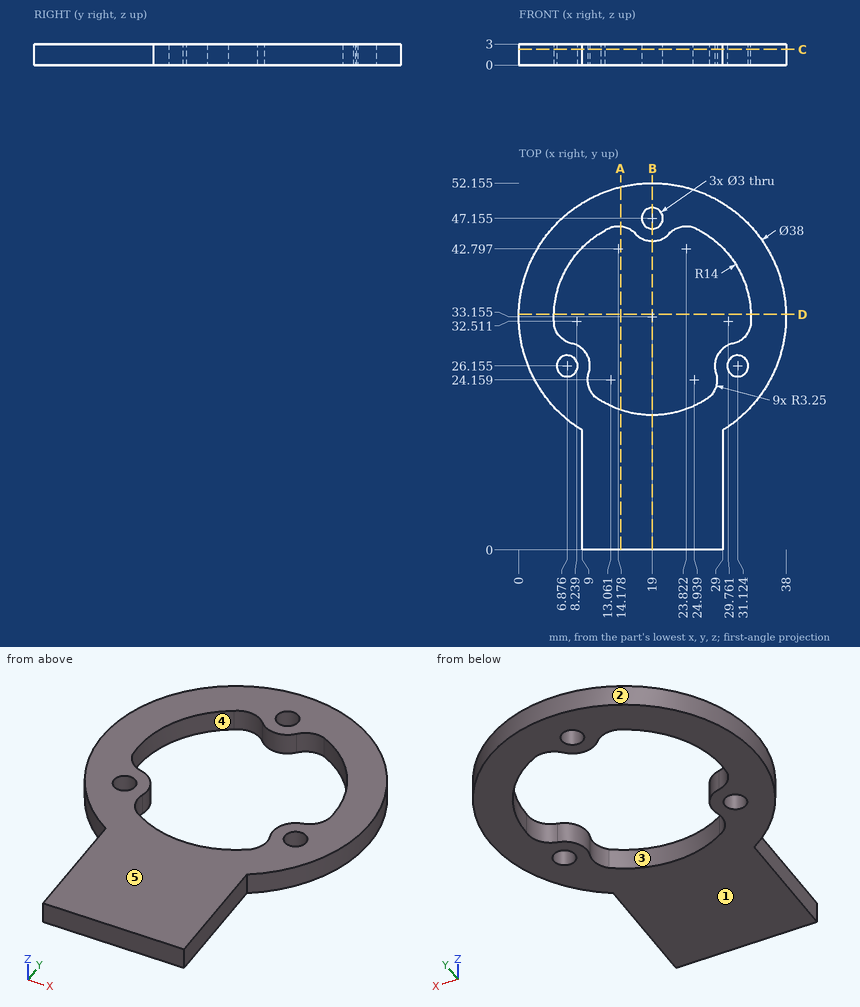
Can you work these out from the drawing? Everything is in mm from the part's minimum corner. A direction names the side the tool comes from. Give positions to 0.01 mm unless a question says otherwise; leave off trailing zeros. Order: outer loops, then holes, each group sorted by start corner. A loop starts at its lowest first (then second) coordinate and runs counter-clockwise, first axis right, second up.
1. Suppose I cut it at C-C (z = 2.25). Give the number of separate pieces and of enclosed holes in the cut face, plus the area to 3 significant figures.
2. Suppose I cut it at A-A (x = 14.5). List the corners of the cut face in (y, z) for me (1 decimal).
3. For the marked faces 4 and 5, which set-ups out of +Z, -Z, +X, -X, +Y, -Y let a thin tool reach every point of the face, with its end or its side?
4. I need wall thicknesses on L1, parallel to Y at x = 19, z = 2.15 (1 decimal); L2, parallel to Y at x = 30.5, z = 1.9 (1 decimal); L3, parallel to X at y = 4, z = 1.2. Which ranges of each line are inside material? Lowest first, please.
5. Suppose I cut it at B-B (x = 19). List the corners of the cut face in (y, z) for me (1 decimal).
6. Will these pins go through, and if not, where does the flat tip stop? P1, Ø1.5, axis at y = 7.5, z = 1.5, coming from the -X side; P2, Ø1.5, axis at y = 4.5, z = 1.5, coming from the +X side; P3, Ø1, axis at x = 14, z = 1.5, coming from the +Y side (1 decimal).
7. We'd pull the mould along X, two halves only. Please class the marked faces 1, 2 and 3: pulls with the +X half, pulls with the -X half, needs draft (parallel to the pull), parting line crosses it, or undercut.
8. Suppose I cut it at D-D (y = 33.5). List the corners of the cut face in (x, z) for me (1 decimal).
Solved:
1. separate pieces: 1
1. enclosed holes: 4
1. area: 854 mm2
2. outline: (0, 0) - (19.9, 0) - (19.9, 3) - (0, 3) - close; (46, 0) - (51.6, 0) - (51.6, 3) - (46, 3) - close
3. face 4: +Z, -Z
3. face 5: +Z, +X, -X, +Y, -Y
4. L1: y = 0 to 19.2, 43.9 to 45.7, 48.7 to 52.2
4. L2: y = 18 to 24.8, 27.5 to 29.3, 41.1 to 48.3
4. L3: x = 9 to 29
5. outline: (0, 0) - (19.2, 0) - (19.2, 3) - (0, 3) - close; (43.9, 0) - (45.7, 0) - (45.7, 3) - (43.9, 3) - close; (48.7, 0) - (52.2, 0) - (52.2, 3) - (48.7, 3) - close
6. P1: stops at x = 9
6. P2: stops at x = 29
6. P3: stops at y = 51.6
7. face 1: needs draft
7. face 2: parting line crosses it
7. face 3: undercut
8. outline: (0, 0) - (5, 0) - (5, 3) - (0, 3) - close; (33, 0) - (38, 0) - (38, 3) - (33, 3) - close
